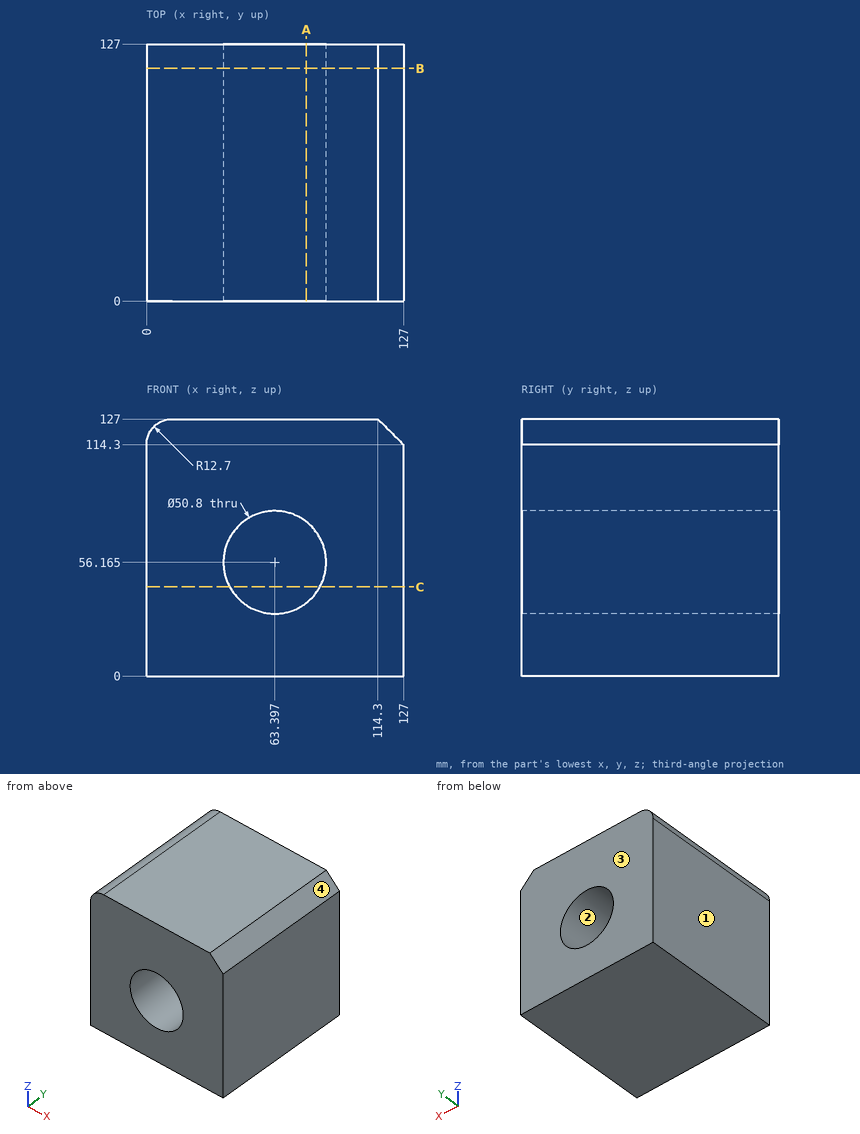
The figure shows three views and two pictorial views of one solid part (mm, origin at its lowest corner). Answer the questions. Give positions to 0.01 mm unless a question says otherwise; leave off trailing zeros. Loops run counter-clockwise (first coordinate to the right, second up) from the corner with the lowest first, then second, coordinate; pieces in that order, holes last. Notation, with made-up numbers: (83.25, 40) -> (107.25, 40) arc R19 cw to (107.25, 77) -> close; hole circle Ø3 at (19, 11). An arc over 180 degrees is marked (long way). Put each result on its own line as item: value. Start each with the question number.
Item 1: The mould has two halves that part along X. Classify the marked faces 1, 2, 3 and 4: released by +X, released by -X, zero draft, split by the parting line, or undercut.
Item 2: The part is cut by section B-B (y = 115). Give the vertices of the cut face in (x, z) (1 decimal).
Item 3: Find the intervals of material crossed by L1, parallel to X at y = 62, z = 53 (1 decimal); L2, parallel to X at y = 78.5, z = 35 (1 decimal); L3, parallel to Z at x = 69, y = 45, in increasing order. Write a range as [from, to].
Item 4: The part is cut by section C-C (z = 44). Give the vertices of the cut face in (x, y) (1 decimal), then the cut area to 3 significant figures.
Item 5: The part is cut by section A-A (x = 79). Give the vertices of the cut face in (y, z).
Answers below:
1. face 1: released by -X
1. face 2: undercut
1. face 3: zero draft
1. face 4: released by +X
2. outline: (0, 0) -> (127, 0) -> (127, 114.3) -> (114.3, 127) -> (12.7, 127) arc R12.7 ccw to (0, 114.3) -> close; hole circle Ø50.8 at (63.4, 56.2)
3. L1: [0, 38.2], [88.6, 127]
3. L2: [0, 49.4], [77.4, 127]
3. L3: [0, 31.39], [80.94, 127]
4. outline: (0, 0) -> (41.1, 0) -> (41.1, 127) -> (0, 127) -> close; (85.7, 0) -> (127, 0) -> (127, 127) -> (85.7, 127) -> close
4. area: 10,500 mm2
5. outline: (0, 0) -> (127, 0) -> (127, 36.12) -> (0, 36.12) -> close; (0, 76.21) -> (127, 76.21) -> (127, 127) -> (0, 127) -> close
